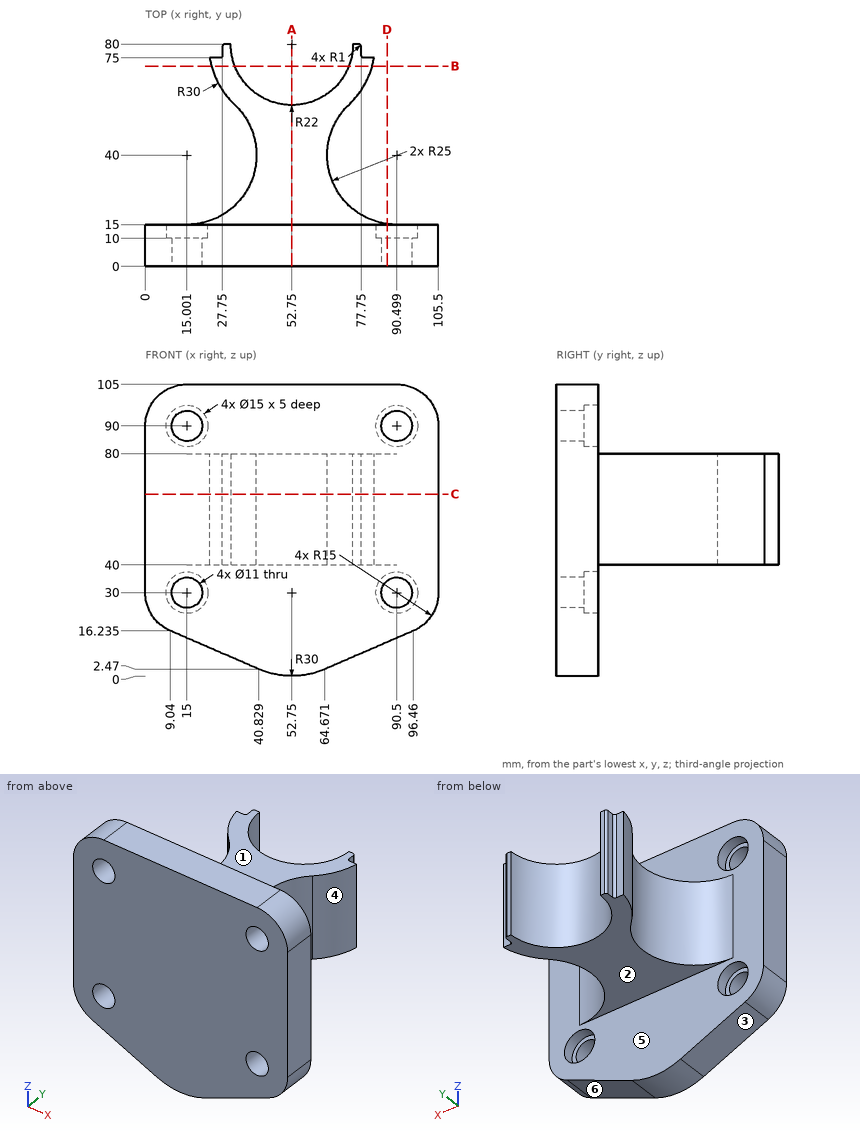
Here's the drawing with two shaded views (mm, measured from the low corner). I have some questions. A direction names the side the tool comes from. Round coordinates to 2 decimals unless told otherwise and drop trailing zeros. Write each loop counter-clockwise with the first axis right and the second up, starting at its lowest first coordinate (ties: lowest second). Pieces come first, ordered by that corner, then holes. Notation, with made-up numbers: M 47,33 L 66,33 A28 cw 66,72 Z; hole C 74.5,41.5 d6. An arc over 180 degrees is marked long. Answer in a Markdown table with one row per item. Add a question column.
Q1. Imagine slicing it at C-C (z = 65.5). Please give me the cut outline in (x, y), then the cut area to 3 significant figures.
Q2. Will these pins go through, and if not, where does the flat tip stop? pin 1 Ø3 at (x, z) = (11, 44) entering from +Y; pin 2 Ø6.5 at (x, z) = (90.5, 90) entering from -Y; pin 3 Ø3.5 at (y, z) = (78, 59) entering from -X; pin 4 Ø6 at (x, z) = (68.5, 51.5) entering from +Y.
Q3. Imagine slicing it at A-A (x = 52.75). Please give me the cut outline in (y, z).
Q4. On a 3-axis mill with a long thin cutter (end or side, diameter ignored), from which of +Z, -Z, +X, -X, +Y, -Y can I reach the whole of each face in a straight line? I mean the marked faces 1, 2 and 3. Say none if no direction works.
Q5. If we mould it in two halves opening along Y, with no side actions, what happens to the marked faces 4, 5 and 6? For each: +Y half, -Y half, draft (parallel to the pull), parting line (faces both ways), or undercut.
Q6. If I drill on line 1 (X direction, y = 12, z = 90); line 2 (X direction, y = 5, z = 90); line 3 (Y direction, x = 27, z = 19), over which ranges is the centre line in solid material (lowest first)? Write a range as from..to.
Q7. Imagine slicing it at B-B (y = 72). Please give me the cut outline in (x, z).
Q8. Imagine slicing it at D-D (x = 87). Please give me the cut outline in (y, z).
Values:
| question | item | result |
|---|---|---|
| 1 | outline | M 0,0 L 105.5,0 L 105.5,15 L 90.5,15 A25 cw 73.34,58.18 A30 ccw 82.33,75 L 78.75,75 A1 cw 77.75,76 L 77.75,79 A1 ccw 76.75,80 L 74.75,80 A22 cw 30.75,80 L 28.75,80 A1 ccw 27.75,79 L 27.75,76 A1 cw 26.75,75 L 23.17,75 A30 ccw 32.16,58.18 A25 cw 15,15 L 0,15 Z |
| 1 | area | 3,410 mm^2 |
| 2 | pin 1 | y = 15 |
| 2 | pin 2 | through |
| 2 | pin 3 | x = 27.75 |
| 2 | pin 4 | y = 68.49 |
| 3 | outline | M 0,0 L 15,0 L 15,40 L 58,40 L 58,80 L 15,80 L 15,105 L 0,105 Z |
| 4 | face 1 | +Z, +X, -X, +Y |
| 4 | face 2 | -Z, +X, -X, +Y |
| 4 | face 3 | -Z, -X, +Y, -Y |
| 5 | face 4 | undercut |
| 5 | face 5 | +Y half |
| 5 | face 6 | draft |
| 6 | line 1 | 0..7.5, 22.5..83, 98..105.5 |
| 6 | line 2 | 0..9.5, 20.5..85, 96..105.5 |
| 6 | line 3 | 0..15 |
| 7 | outline | M 23.84,40 L 32.26,40 L 32.26,80 L 23.84,80 Z; M 73.24,40 L 81.66,40 L 81.66,80 L 73.24,80 Z |
| 8 | outline | M 0,12.14 L 15,12.14 L 15,23.37 L 10,23.37 L 10,25.76 L 0,25.76 Z; M 0,34.24 L 10,34.24 L 10,36.63 L 15,36.63 L 15,40 L 15.25,40 L 15.25,80 L 15,80 L 15,83.37 L 10,83.37 L 10,85.76 L 0,85.76 Z; M 0,94.24 L 10,94.24 L 10,96.63 L 15,96.63 L 15,105 L 0,105 Z |
